```python
from build123d import *

# Parameters (mm, degrees)
F0_W     = 110
F0_H     = 60
F0_R     = 3.25
F0_R_2   = 3.3
F0_R_3   = 3
F0_R_4   = 3.05
F0_R_5   = 3.1
F0_R_6   = 3.15
F0_R_7   = 3.2
F0_R_8   = 1.85
F0_R_9   = 1.5
F0_R_10  = 1.9
F0_R_11  = 1.95
F0_R_12  = 1.55
F0_R_13  = 1.6
F0_R_14  = 2
F0_R_15  = 2.05
F0_R_16  = 1.65
F0_R_17  = 1.7
F0_R_18  = 1.75
F0_R_19  = 2.1
F0_W_2   = 5.055394
F0_H_2   = 31.174931
F1_DEPTH = 10


with BuildPart() as f1:
    # F0 (on Top) → F1 (new body)
    with BuildSketch(Plane.XY):
        Rectangle(F0_W, F0_H)
        with Locations((-29.181362, -20.761674)):
            Circle(F0_R, mode=Mode.SUBTRACT)
        with Locations((-9.345621, -20.652689)):
            Circle(F0_R_2, mode=Mode.SUBTRACT)
        with Locations((-36.208221, -9.176929)):
            Circle(F0_R_3, mode=Mode.SUBTRACT)
        with Locations((-18.724983, -9.808854)):
            Circle(F0_R_4, mode=Mode.SUBTRACT)
        with Locations((-1.873668, -10.124817)):
            Circle(F0_R_5, mode=Mode.SUBTRACT)
        with Locations((13.819118, -10.335458)):
            Circle(F0_R_6, mode=Mode.SUBTRACT)
        with Locations((30.455841, -11.228606)):
            Circle(F0_R_7, mode=Mode.SUBTRACT)
        with Locations((-38.841237, 1.1445)):
            Circle(F0_R_8, mode=Mode.SUBTRACT)
        with Locations((-37.156106, 11.676571)):
            Circle(F0_R_9, mode=Mode.SUBTRACT)
        with Locations((-23.253773, 0.828538)):
            Circle(F0_R_10, mode=Mode.SUBTRACT)
        with Locations((-9.56208, 0.723217)):
            Circle(F0_R_11, mode=Mode.SUBTRACT)
        with Locations((-24.412301, 11.781892)):
            Circle(F0_R_12, mode=Mode.SUBTRACT)
        with Locations((-10.404645, 11.360609)):
            Circle(F0_R_13, mode=Mode.SUBTRACT)
        with Locations((-39.683805, 21.155436)):
            Circle(F0_R_9, mode=Mode.SUBTRACT)
        with Locations((-25.044224, 21.366077)):
            Circle(F0_R_12, mode=Mode.SUBTRACT)
        with Locations((-10.931249, 21.471397)):
            Circle(F0_R_13, mode=Mode.SUBTRACT)
        with Locations((5.604102, 0.407255)):
            Circle(F0_R_14, mode=Mode.SUBTRACT)
        with Locations((18.979832, 1.1445)):
            Circle(F0_R_15, mode=Mode.SUBTRACT)
        with Locations((0, 11.992533)):
            Circle(F0_R_16, mode=Mode.SUBTRACT)
        with Locations((13.819118, 11.887213)):
            Circle(F0_R_17, mode=Mode.SUBTRACT)
        with Locations((26.878885, 12.308496)):
            Circle(F0_R_18, mode=Mode.SUBTRACT)
        with Locations((32.039602, 1.1445)):
            Circle(F0_R_19, mode=Mode.SUBTRACT)
        with Locations((45.093073, 4.44514)):
            Rectangle(F0_W_2, F0_H_2, mode=Mode.SUBTRACT)
        with Locations((0, 21.471397)):
            Circle(F0_R_16, mode=Mode.SUBTRACT)
        with Locations((13.187193, 21.471397)):
            Circle(F0_R_17, mode=Mode.SUBTRACT)
        with Locations((26.562924, 21.471397)):
            Circle(F0_R_18, mode=Mode.SUBTRACT)
    extrude(amount=F1_DEPTH)


solid = f1.part
```
Geometry check sheet. Reference: the model listing, model coordinates, mm. A direction names the side the tool comes from. Coordinates: 2 decimals unless noted, no trailing zeros. Order: outer loops, then holes, each group sorted by start corner. A loop starts at its lowest first (then second) coordinate and runs counter-clockwise, first axis right, second up. Notation, with made-up numbers: (29.25, 73) - (62.25, 73) arc R22 ccw to (62.25, 100) - close; hole circle Ø2 at (-2, -14). An arc over 180 degrees is marked (long way). Answer in a Markdown table with one row per item. Add a question column.
1. Section check C-C (x = 0). Enter the section's corners in (y, z).
2. Section check A-A (x = 32.5). Enter the section's corners in (y, z), plus the area to 3 significant figures.
3. Material ranges on L1, parallel to X at y = 4, z = 8.25; L2, parallel to Y at x = 32, z = 9; L3, parallel to X at y = -20, z = 7, recorded low to high. Write a range as [from, to].
4. Section check B-B (z = 8.5). Give the number of separate pieces and of enclosed holes in the cut face, plus the area to 3 significant figures.
5. Draft check along X on faces 1 (the face through (55, 0, 5)), 2 (the face through (-55, 0, 5)), 3 (the face through (45, 20.033, 5)). Enter one of: +X half, -X half, draft (parallel to the pull), parting line (faces both ways), or undercut.
6. Access from +Z, -Z, +X, -X, +Y, -Y to the whole of each face (thin tool, end or side, straight path). Record for faces 4 (the face through (-1, 30, 5)), 5 (the face through (45, -11.142, 5)).
Data:
| question | item | result |
|---|---|---|
| 1 | outline | (-30, 0) - (-12.59, 0) - (-12.59, 10) - (-30, 10) - close; (-7.66, 0) - (10.34, 0) - (10.34, 10) - (-7.66, 10) - close; (13.64, 0) - (19.82, 0) - (19.82, 10) - (13.64, 10) - close; (23.12, 0) - (30, 0) - (30, 10) - (23.12, 10) - close |
| 2 | outline | (-30, 0) - (-13.69, 0) - (-13.69, 10) - (-30, 10) - close; (-8.77, 0) - (-0.9, 0) - (-0.9, 10) - (-8.77, 10) - close; (3.19, 0) - (30, 0) - (30, 10) - (3.19, 10) - close |
| 2 | area | 510 mm² |
| 3 | L1 | x = [-55, 42.57], [47.62, 55] |
| 3 | L2 | y = [-30, -14.03], [-8.43, -0.96], [3.24, 30] |
| 3 | L3 | x = [-55, -32.34], [-26.02, -12.58], [-6.11, 55] |
| 4 | separate pieces | 1 |
| 4 | enclosed holes | 26 |
| 4 | area | 6,050 mm² |
| 5 | face 1 | +X half |
| 5 | face 2 | -X half |
| 5 | face 3 | undercut |
| 6 | face 4 | +Z, -Z, +X, -X, +Y |
| 6 | face 5 | +Z, -Z |
